```python
from build123d import *

# Parameters (mm, degrees)
SKETCH1_R             = 15.875
BOSS_EXTRUDE1_DEPTH   = 10
FILLET1_R             = 1
F_4_CLEARANCE_HOLE1_D = 3.2639


with BuildPart() as part:
    # Sketch1 → Boss-Extrude1 (new body)
    with BuildSketch(Plane.XY):
        with BuildLine():
            Line((-20.875, 0), (-20.875, -20))
            Line((-20.875, -20), (-32.875, -20))
            Line((-32.875, -20), (-32.875, -23.72))
            Line((-32.875, -23.72), (32.875, -23.72))
            Line((32.875, -23.72), (32.875, -20))
            Line((32.875, -20), (20.875, -20))
            Line((20.875, -20), (20.875, 0))
            ThreePointArc((20.875, 0), (0, 20.875), (-20.875, 0))
        make_face()
        Circle(SKETCH1_R, mode=Mode.SUBTRACT)
    extrude(amount=BOSS_EXTRUDE1_DEPTH)

    # Fillet1
    fillet1_edges = [part.edges().sort_by_distance(p)[0] for p in [
        (-32.875, -21.86, 10),
        (32.875, -21.86, 10),
        (32.875, -21.86, 0),
        (-32.875, -21.86, 0),
    ]]
    fillet(fillet1_edges, radius=FILLET1_R)

    # #4 Clearance Hole1 (through all)
    with Locations(Plane(origin=(0, -20, 0), x_dir=(1, 0, 0), z_dir=(0, 1, 0))):
        with Locations((-26.875, -5), (26.875, -5)):
            Hole(F_4_CLEARANCE_HOLE1_D / 2)


solid = part.part
```
Geometry: final body of the model. Coordinates: model frame, mm. A direction names the side the tool comes from. Round coordinates to 2 decimals unless told otherwise and drop trailing zeros. Loops run counter-clockwise (first coordinate to the right, second up) from the corner with the lowest first, then second, coordinate; pieces in that order, holes last.
Item 1: Reachability of faces 5 (the cylindrical face through (25.32, -21.89, 4.51)), 6 (the flat face through (28.3, -20, 3.8)), 7 (the flat face through (-25, -20, 4)) from +Z, -Z, +X, -X, +Y, -Y: full face, straight path, thin tool, end or side. Return the list, or none.
Checked values:
face 5: +Y, -Y
face 6: +Z, -Z, +X, +Y
face 7: +Z, -Z, -X, +Y
Item 2: Mould query, pull axis Z, two halves, no side actions, for faces 1 (the flat face through (20.875, -10, 5)), 2 (the cylindrical face through (-25.245, -21.886, 4.928)), 3 (the flat face through (-0.1, -16.2, 0)), 4 (the flat face through (-0.1, -16.2, 10)). Classes: released by +Z, released by -Z, zero draft, split by the parting line, or undercut.
Checked values:
face 1: zero draft
face 2: undercut
face 3: released by -Z
face 4: released by +Z
Item 3: Section C-C, the plane z = 8.25. Output: boundary loops of the cut face in (x, y) (3 decimals), plus the area to 3 significant figures.
Checked values:
outline: (-32.875, -23.72) - (32.875, -23.72) - (32.875, -20) - (20.875, -20) - (20.875, 0) arc R20.875 ccw to (-20.875, 0) - (-20.875, -20) - (-32.875, -20) - close; hole circle Ø31.75 at (0, 0)
area: 972 mm2
Item 4: Contact query for flat-ended pins moving along their axis: P1, Ø5, axis at x = 28, z = 5.5, coming from the +Y side; P2, Ø5, axis at y = -6.5, z = 4.5, coming from the +X side (3 decimals); P3, Ø4, axis at x = -26.875, z = 5, coming from the -Y side. Output: stop coordinate, or through.
Checked values:
P1: stops at y = -20
P2: stops at x = 20.875
P3: stops at y = -23.72
Item 5: Section A-A, the plane z = 5. Output: boundary loops of the cut face in (x, y) (3 decimals), plus the area to 3 significant figures.
Checked values:
outline: (-32.875, -23.72) - (-28.507, -23.72) - (-28.507, -20) - (-32.875, -20) - close; (-25.243, -23.72) - (25.243, -23.72) - (25.243, -20) - (20.875, -20) - (20.875, 0) arc R20.875 ccw to (-20.875, 0) - (-20.875, -20) - (-25.243, -20) - close; (28.507, -23.72) - (32.875, -23.72) - (32.875, -20) - (28.507, -20) - close; hole circle Ø31.75 at (0, 0)
area: 948 mm2
Item 6: Section D-D, the plane y = 4. Output: boundary loops of the cut face in (x, z).
Checked values:
outline: (-20.49, 0) - (-15.36, 0) - (-15.36, 10) - (-20.49, 10) - close; (15.36, 0) - (20.49, 0) - (20.49, 10) - (15.36, 10) - close
Item 7: Line query: L1, parallel to X at y = -22.65, z = 5 (3 decimals); L2, parallel to Y at x = 0, z = 3.25 (3 decimals); L3, parallel to Y at x = -24, z = 5.75. Output: solid intervals per line, ascending.
Checked values:
L1: x = -32.875 to -28.507, -25.243 to 25.243, 28.507 to 32.875
L2: y = -23.72 to -15.875, 15.875 to 20.875
L3: y = -23.72 to -20
Item 8: Section B-B, the plane x = 0. Output: boundary loops of the cut face in (y, z) (3 decimals).
Checked values:
outline: (-23.72, 0) - (-15.875, 0) - (-15.875, 10) - (-23.72, 10) - close; (15.875, 0) - (20.875, 0) - (20.875, 10) - (15.875, 10) - close
